```python
from build123d import *

# Parameters (mm, degrees)
SKETCH1_W                       = 40
SKETCH1_H                       = 90
BOSS_EXTRUDE1_DEPTH             = 9
SKETCH2_W                       = 9
SKETCH2_H                       = 50
BOSS_EXTRUDE2_DEPTH             = 40
BOSS_EXTRUDE3_DEPTH             = 35
SKETCH4_W                       = 35
SKETCH4_H                       = 8.25
BOSS_EXTRUDE4_DEPTH             = 10
SKETCH5_W                       = 35
SKETCH5_H                       = 46.2
BOSS_EXTRUDE5_DEPTH             = 8
SKETCH6_W                       = 35
SKETCH6_H                       = 46.2
BOSS_EXTRUDE6_DEPTH             = 8
SKETCH10_R                      = 2
CUT_EXTRUDE1_DEPTH              = 62.75
CUT_EXTRUDE1_DEPTH_BACK         = 29.25
SKETCH11_R                      = 4.25
CUT_EXTRUDE2_DEPTH              = 4
SKETCH12_R                      = 4.25
CUT_EXTRUDE3_DEPTH              = 4
SKETCH13_W                      = 8
SKETCH13_H                      = 4
CUT_EXTRUDE4_DEPTH              = 47.2
FILLET1_R                       = 4
CUT_EXTRUDE5_DEPTH              = 3
CUT_EXTRUDE6_DEPTH              = 3
SKETCH18_R                      = 1.75
CUT_EXTRUDE7_DEPTH              = 10
SKETCH19_W                      = 40
SKETCH19_H                      = 9
CUT_EXTRUDE8_DEPTH              = 12
SKETCH20_W                      = 40
SKETCH20_H                      = 9
CUT_EXTRUDE9_DEPTH              = 12
CUT_EXTRUDE10_REACH             = 18.25
SKETCH21_W                      = 8.5
SKETCH21_H                      = 5
CUT_EXTRUDE10_DIRECTION_2_REACH = 51.75
SKETCH22_W                      = 8
SKETCH22_H                      = 4
CUT_EXTRUDE11_DEPTH             = 14
CUT_EXTRUDE12_DEPTH             = 4
CUT_EXTRUDE12_DEPTH_BACK        = 4
SKETCH25_W                      = 40
SKETCH25_H                      = 9
CUT_EXTRUDE13_DEPTH             = 3
SKETCH26_W                      = 40
SKETCH26_H                      = 9
CUT_EXTRUDE14_DEPTH             = 3


with BuildPart() as part:
    # Sketch1 → Boss-Extrude1 (new body)
    with BuildSketch(Plane.XY):
        with Locations((-17, 0)):
            Rectangle(SKETCH1_W, SKETCH1_H)
    extrude(amount=BOSS_EXTRUDE1_DEPTH)

    # Sketch2 → Boss-Extrude2 (add)
    with BuildSketch(Plane.ZY.offset(37)):
        with Locations((4.5, 0)):
            Rectangle(SKETCH2_W, SKETCH2_H)
    extrude(amount=BOSS_EXTRUDE2_DEPTH)

    # Sketch3 → Boss-Extrude3 (add)
    with BuildSketch(Plane.ZY.offset(77)):
        with BuildLine():
            Line((0, -25), (0, 25))
            Line((0, 25), (-27.2, 25))
            Line((-27.2, 25), (-27.2, 16.75))
            ThreePointArc((-27.2, 16.75), (-15.355961415, 11.844038585), (-10.45, 0))
            ThreePointArc((-10.45, 0), (-15.355961415, -11.844038585), (-27.2, -16.75))
            Line((-27.2, -16.75), (-27.2, -25))
            Line((-27.2, -25), (0, -25))
        make_face()
    extrude(amount=-BOSS_EXTRUDE3_DEPTH)

    # Sketch4 → Boss-Extrude4 (add)
    with BuildSketch(Plane(origin=(0, 0, -27.2), x_dir=(-1, 0, 0), z_dir=(0, 0, -1))):
        with Locations((59.5, -20.875)):
            Rectangle(SKETCH4_W, SKETCH4_H)
        with Locations((59.5, 20.875)):
            Rectangle(SKETCH4_W, SKETCH4_H)
    extrude(amount=BOSS_EXTRUDE4_DEPTH)

    # Sketch5 → Boss-Extrude5 (add)
    with BuildSketch(Plane.XZ.offset(25)):
        with Locations((-59.5, -14.1)):
            Rectangle(SKETCH5_W, SKETCH5_H)
    extrude(amount=BOSS_EXTRUDE5_DEPTH)

    # Sketch6 → Boss-Extrude6 (add)
    with BuildSketch(Plane(origin=(0, 25, 0), x_dir=(1, 0, 0), z_dir=(0, 1, 0))):
        with Locations((-59.5, 14.1)):
            Rectangle(SKETCH6_W, SKETCH6_H)
    extrude(amount=BOSS_EXTRUDE6_DEPTH)

    # Sketch10 → Cut-Extrude1 (cut, two sides)
    with BuildSketch(Plane(origin=(0, -16.75, 0), x_dir=(1, 0, 0), z_dir=(0, 1, 0))) as cut_extrude1_sk:
        with Locations((-59.5, 32.2)):
            Circle(SKETCH10_R)
    extrude(amount=CUT_EXTRUDE1_DEPTH, mode=Mode.SUBTRACT)
    extrude(cut_extrude1_sk.sketch, amount=-CUT_EXTRUDE1_DEPTH_BACK, mode=Mode.SUBTRACT)

    # Sketch11 → Cut-Extrude2 (cut)
    with BuildSketch(Plane(origin=(0, -16.75, 0), x_dir=(1, 0, 0), z_dir=(0, 1, 0))):
        with Locations((-59.5, 32.2)):
            Circle(SKETCH11_R)
    extrude(amount=-CUT_EXTRUDE2_DEPTH, mode=Mode.SUBTRACT)

    # Sketch12 → Cut-Extrude3 (cut)
    with BuildSketch(Plane.XZ.offset(-16.75)):
        with Locations((-59.5, -32.2)):
            Circle(SKETCH12_R)
    extrude(amount=-CUT_EXTRUDE3_DEPTH, mode=Mode.SUBTRACT)

    # Sketch13 → Cut-Extrude4 (cut, through all)
    with BuildSketch(Plane(origin=(0, 0, -37.2), x_dir=(-1, 0, 0), z_dir=(0, 0, -1))):
        with Locations((50, 24.875)):
            Rectangle(SKETCH13_W, SKETCH13_H)
        with Locations((69, 24.875)):
            Rectangle(SKETCH13_W, SKETCH13_H)
        with Locations((50, -24.875)):
            Rectangle(SKETCH13_W, SKETCH13_H)
        with Locations((69, -24.875)):
            Rectangle(SKETCH13_W, SKETCH13_H)
    extrude(amount=-CUT_EXTRUDE4_DEPTH, mode=Mode.SUBTRACT)

    # Fillet1
    fillet1_edges = [part.edges().sort_by_distance(p)[0] for p in [
        (-69, 22.875, -37.2),
        (-50, -22.875, -37.2),
        (-69, -22.875, -37.2),
        (-50, 22.875, -37.2),
    ]]
    fillet(fillet1_edges, radius=FILLET1_R)

    # Sketch16 → Cut-Extrude5 (cut)
    with BuildSketch(Plane.XZ.offset(33)):
        Polygon((-57.421539031, -28.6), (-61.578460969, -28.6), (-63.656921938, -32.2), (-61.578460969, -35.8), (-57.421539031, -35.8), (-55.343078062, -32.2), align=None)
    extrude(amount=-CUT_EXTRUDE5_DEPTH, mode=Mode.SUBTRACT)

    # Sketch17 → Cut-Extrude6 (cut)
    with BuildSketch(Plane(origin=(0, 33, 0), x_dir=(1, 0, 0), z_dir=(0, 1, 0))):
        Polygon((-61.578460969, 28.6), (-57.421539031, 28.6), (-55.343078062, 32.2), (-57.421539031, 35.8), (-61.578460969, 35.8), (-63.656921938, 32.2), align=None)
    extrude(amount=-CUT_EXTRUDE6_DEPTH, mode=Mode.SUBTRACT)

    # Sketch18 → Cut-Extrude7 (cut)
    with BuildSketch(Plane(origin=(0, 0, 0), x_dir=(-1, 0, 0), z_dir=(0, 0, -1))):
        with Locations((5.45, 15.05)):
            Circle(SKETCH18_R)
        with Locations((5.45, -15.05)):
            Circle(SKETCH18_R)
        with Locations((29.55, -15.05)):
            Circle(SKETCH18_R)
        with Locations((29.55, 15.05)):
            Circle(SKETCH18_R)
    extrude(amount=-CUT_EXTRUDE7_DEPTH, mode=Mode.SUBTRACT)

    # Sketch19 → Cut-Extrude8 (cut)
    with BuildSketch(Plane(origin=(0, 45, 0), x_dir=(1, 0, 0), z_dir=(0, 1, 0))):
        with Locations((-17, -4.5)):
            Rectangle(SKETCH19_W, SKETCH19_H)
    extrude(amount=-CUT_EXTRUDE8_DEPTH, mode=Mode.SUBTRACT)

    # Sketch20 → Cut-Extrude9 (cut)
    with BuildSketch(Plane.XZ.offset(45)):
        with Locations((-17, 4.5)):
            Rectangle(SKETCH20_W, SKETCH20_H)
    extrude(amount=-CUT_EXTRUDE9_DEPTH, mode=Mode.SUBTRACT)

    # Cut-Extrude10: up to this face of the body (flat: up to its plane)
    cut_extrude10_end = Plane(part.part.faces().sort_by_distance((-63.629791847, -20.75, -32.2))[0])
    # Sketch21 → Cut-Extrude10 (cut, up to the picked face)
    with BuildSketch(Plane(origin=(0, -16.75, 0), x_dir=(1, 0, 0), z_dir=(0, 1, 0)), mode=Mode.PRIVATE) as cut_extrude10_sk1:
        with Locations((-59.5, 34.7)):
            Rectangle(SKETCH21_W, SKETCH21_H)
    cut_extrude10_tool1 = split(extrude(cut_extrude10_sk1.sketch, amount=-CUT_EXTRUDE10_REACH, mode=Mode.PRIVATE), bisect_by=cut_extrude10_end, keep=Keep.BOTH, mode=Mode.PRIVATE)
    add(cut_extrude10_tool1.solids().sort_by_distance((-59.5, -16.75, -34.7))[0], mode=Mode.SUBTRACT)

    # Cut-Extrude10 direction 2: up to this face of the body (flat: up to its plane)
    cut_extrude10_direction_2_end = Plane(part.part.faces().sort_by_distance((-63.629791847, 20.75, -32.2))[0])
    # Sketch21 → Cut-Extrude10 direction 2 (cut, up to the picked face)
    with BuildSketch(Plane(origin=(0, -16.75, 0), x_dir=(1, 0, 0), z_dir=(0, 1, 0)), mode=Mode.PRIVATE) as cut_extrude10_direction_2_sk1:
        with Locations((-59.5, 34.7)):
            Rectangle(SKETCH21_W, SKETCH21_H)
    cut_extrude10_direction_2_tool1 = split(extrude(cut_extrude10_direction_2_sk1.sketch, amount=CUT_EXTRUDE10_DIRECTION_2_REACH, mode=Mode.PRIVATE), bisect_by=cut_extrude10_direction_2_end, keep=Keep.BOTH, mode=Mode.PRIVATE)
    add(cut_extrude10_direction_2_tool1.solids().sort_by_distance((-59.5, -16.75, -34.7))[0], mode=Mode.SUBTRACT)

    # Sketch22 → Cut-Extrude11 (cut)
    with BuildSketch(Plane.XY.offset(9)):
        with Locations((-19.773502692, -23.75)):
            Rectangle(SKETCH22_W, SKETCH22_H)
        with Locations((-19.773502692, 23.75)):
            Rectangle(SKETCH22_W, SKETCH22_H)
    extrude(amount=-CUT_EXTRUDE11_DEPTH, mode=Mode.SUBTRACT)

    # Sketch23 → Cut-Extrude12 (cut, two sides)
    with BuildSketch(Plane(origin=(0, 0, 0), x_dir=(1, 0, 0), z_dir=(0, 1, 0))) as cut_extrude12_sk:
        with BuildLine():
            ThreePointArc((-69, -9), (-71.343145751, -3.343145751), (-77, -1))
            Line((-77, -1), (-77, -4))
            ThreePointArc((-77, -4), (-73.464466094, -5.464466094), (-72, -9))
            Line((-72, -9), (-69, -9))
        make_face()
        with BuildLine():
            Line((-77, -4), (-77, -1))
            ThreePointArc((-77, -1), (-82.656854249, -14.656854249), (-69, -9))
            Line((-69, -9), (-72, -9))
            ThreePointArc((-72, -9), (-80.535533906, -12.535533906), (-77, -4))
        make_face()
    extrude(amount=CUT_EXTRUDE12_DEPTH, mode=Mode.SUBTRACT)
    extrude(cut_extrude12_sk.sketch, amount=-CUT_EXTRUDE12_DEPTH_BACK, mode=Mode.SUBTRACT)

    # Sketch25 → Cut-Extrude13 (cut)
    with BuildSketch(Plane(origin=(0, 33, 0), x_dir=(1, 0, 0), z_dir=(0, 1, 0))):
        with Locations((-17, -4.5)):
            Rectangle(SKETCH25_W, SKETCH25_H)
    extrude(amount=-CUT_EXTRUDE13_DEPTH, mode=Mode.SUBTRACT)

    # Sketch26 → Cut-Extrude14 (cut)
    with BuildSketch(Plane.XZ.offset(33)):
        with Locations((-17, 4.5)):
            Rectangle(SKETCH26_W, SKETCH26_H)
    extrude(amount=-CUT_EXTRUDE14_DEPTH, mode=Mode.SUBTRACT)


solid = part.part
```
CAD build for the part. Positions are in the model's coordinates, mm. A direction names the side the tool comes from. Coordinates: 2 decimals unless noted, no trailing zeros. Write each loop counter-clockwise with the first axis right and the second up, starting at its lowest first coordinate (ties: lowest second). Pieces come first, ordered by that corner, then holes. Notation, with made-up numbers: (4, -10) -> (41, -10) arc R14 cw to (41, 12) -> close; hole circle Ø2 at (-39.5, 32.25). An arc over 180 degrees is marked (long way). Return JSON: item names as keys, results as strings. Group by question number.
Q1. Cut at D-D, the plane y = 15.05. Give the cut face in (x, z), then the cut area to 3 significant figures.
Q2. Pull direction Y, two halves, no side cores. Call faces 6 (the face through (-62.6, -31.52, -30.37)), 7 (the face through (-63.75, -19, -35)), 8 (the face through (-40, 25, 5)), 9 (the face through (-73, -4, 5)): released by +Y, released by -Y, zero draft, split by the parting line, or undercut.
Q3. Drill centre lines: line 1 (Y direction, x = -29.55, z = 5.25); line 2 (X direction, y = 26, z = -4); line 3 (X direction, y = 15, z = 6). Where is each one in solid material? Low to high.
Q4. Which spindle directions (+Z, -Z, +X, -X, +Y, -Y) get a long thin tool onto all of the face, cutting with end or side? Do faces 1 (the face through (-73, 4, 5)), 2 (the face through (-39, -25, 5)), 3 (the face through (-69, -26.875, -14)), 4 (the face through (-56.368, 31.521, -33.975)), 5 (the face through (-59, -32, -28.6)). Say none if no direction does.
Q5. Cut at B-B, the plane x = -59.5. Give the cut face in (y, z), then the cut area to 3 significant figures.
Q6. Cut at C-C, the plane z = -1. Give the cut face in (x, y) (3 decimals).
Q7. Cut at A-A, the plane y = -24. Give the cut face in (x, z).
Q8. Flat gauge pins, fed straight in: pin 1 (12 mm diameter, centred on y = 23, z = -15.5, fed in from +X); pin 2 (2 mm diameter, centred on x = -61, z = -32.5, fed in from -Y); pin 3 (5.5 mm diameter, centred on x = -39, z = 3.5, fed in from +Y). Where does each tip first touch, or does it go through?
Returned:
{
 "1": {"outline": "(-77, -19.85) -> (-42, -19.85) -> (-42, 0) -> (-31.3, 0) -> (-31.3, 9) -> (-77, 9) -> close; (-27.8, 0) -> (-7.2, 0) -> (-7.2, 9) -> (-27.8, 9) -> close; (-3.7, 0) -> (3, 0) -> (3, 9) -> (-3.7, 9) -> close", "area": "1,350 mm2"},
 "2": {"face 6": "zero draft", "face 7": "undercut", "face 8": "released by +Y", "face 9": "undercut"},
 "3": {"line 1": "y = -30 to -16.8, -13.3 to 13.3, 16.8 to 30", "line 2": "x = -77 to -73, -65 to -54, -46 to -42", "line 3": "x = -77 to -31.3, -27.8 to -7.2, -3.7 to 3"},
 "4": {"face 1": "none", "face 2": "+Z, -Z, -Y", "face 3": "+Z, -Z", "face 4": "+Y", "face 5": "-Y"},
 "5": {"outline": "(-33, -37.2) -> (-20.75, -37.2) -> (-20.75, -34.2) -> (-30, -34.2) -> (-30, -35.8) -> (-33, -35.8) -> close; (-33, -28.6) -> (-30, -28.6) -> (-30, -30.2) -> (-20.75, -30.2) -> (-20.75, -27.95) -> (-16.75, -27.95) -> (-16.75, -27.2) arc R16.75 cw to (16.75, -27.2) -> (16.75, -27.95) -> (20.75, -27.95) -> (20.75, -30.2) -> (30, -30.2) -> (30, -28.6) -> (33, -28.6) -> (33, 9) -> (-33, 9) -> close; (20.75, -37.2) -> (33, -37.2) -> (33, -35.8) -> (30, -35.8) -> (30, -34.2) -> (20.75, -34.2) -> close", "area": "2,080 mm2"},
 "6": {"outline": "(-77, -33) -> (-42, -33) -> (-42, 33) -> (-77, 33) -> close; hole (-73, -26.875) -> (-65, -26.875) -> (-65, -22.875) -> (-73, -22.875) -> close; hole (-73, 22.875) -> (-65, 22.875) -> (-65, 26.875) -> (-73, 26.875) -> close; hole (-54, -26.875) -> (-46, -26.875) -> (-46, -22.875) -> (-54, -22.875) -> close; hole (-54, 22.875) -> (-46, 22.875) -> (-46, 26.875) -> (-54, 26.875) -> close"},
 "7": {"outline": "(-77, -37.2) -> (-73, -37.2) -> (-73, 9) -> (-77, 9) -> close; (-65, -37.2) -> (-54, -37.2) -> (-54, 9) -> (-65, 9) -> close; (-46, -37.2) -> (-42, -37.2) -> (-42, 0) -> (-23.77, 0) -> (-23.77, 9) -> (-46, 9) -> close; (-15.77, 0) -> (3, 0) -> (3, 9) -> (-15.77, 9) -> close; hole circle Ø4 at (-59.5, -32.2)"},
 "8": {"pin 1": "stops at x = -42", "pin 2": "stops at y = -30", "pin 3": "stops at y = 30"}
}
